The listing builds one solid part. Answer for the finished solid, in the listing's coordinates (mm). Give positions to 0.01 mm unless a question says otherwise; leave off trailing zeros. Order: outer loops, then holes, each group sorted by start corner. A loop starts at its lowest first (then second) coordinate and runs counter-clockwise, first axis right, second up. Notation, with made-up numbers: (43.25, 80) - (88.25, 80) arc R15 cw to (88.25, 95) - close; hole circle Ø6 at (-6, 14). An arc over 180 degrees is marked (long way). Use a Markdown table: item, result. Add a question column.
1) Straight lines are drawn through the part: line 1 (X direction, y = 1.75, z = 2.25); line 2 (Z direction, x = -20, y = 0.25); line 3 (Y direction, x = -0.5, z = -0.1). For each, find the intervals that lie inside material, in ascending order.
2) Find section A-A, the plane y = 13. Determine the outline of the cut face in (x, z).
3) Flat-ended cylindrical pins translate along their axes: pin 1 (0.9 mm diameter, centred on x = 15, z = 2, fed in from -Y); pin 2 (0.7 mm diameter, centred on y = 0, z = 2, fed in from +X); pin 3 (12 mm diameter, centred on x = -3, y = -4, fed in from +Z); pin 4 (1.5 mm diameter, centred on x = 11.5, z = 1, fed in from +Y). Find the tip coordinate at first contact, or state that the pin passes through.
4) Find section B-B, the plane x = -7. Determine the outline of the cut face in (y, z), plus the area to 3 significant figures.
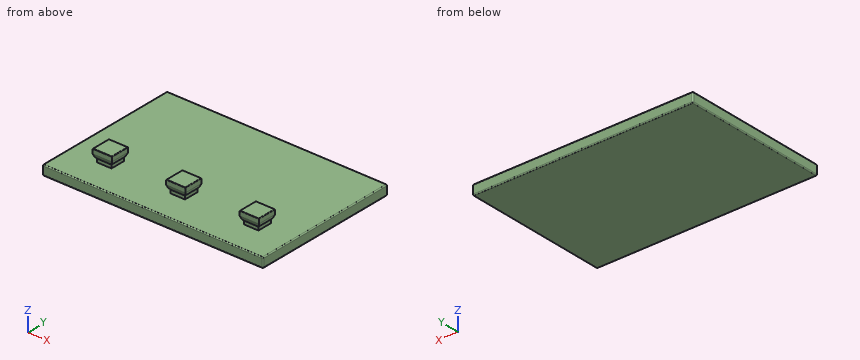
from build123d import *

# Parameters (mm, degrees)
SKETCH_1_W          = 45
SKETCH_1_H          = 30
EXTRUDE_1_DEPTH     = 2
SKETCH_2_W          = 3
SKETCH_2_H          = 3
EXTRUDE_2_DEPTH     = 1
EXTRUDE_START       = -4
EXTRUDE_3_DEPTH     = 5
CUT_EXTRUDE_1_REACH = 35.321
FILLET_1_R          = 0.1
FILLET_2_R          = 0.2


with BuildPart() as part:
    # Sketch 1 → Extrude 1 (new body)
    with BuildSketch(Plane.XY):
        with Locations((0, 7.5)):
            Rectangle(SKETCH_1_W, SKETCH_1_H)
    extrude(amount=-EXTRUDE_1_DEPTH)

    # Sketch 2 → Extrude 2 (add)
    with BuildSketch(Plane.XY):
        Rectangle(SKETCH_2_W, SKETCH_2_H)
    extrude_2 = extrude(amount=EXTRUDE_2_DEPTH)

    # Sketch 3 → Extrude 3 (add)
    with BuildSketch(Plane.XZ.offset(1.5).offset(EXTRUDE_START)):
        with BuildLine():
            Line((-1.95, 2.5), (1.95, 2.5))
            Line((1.95, 2.5), (1.95, 1.555590279))
            ThreePointArc((1.95, 1.555590279), (1.780042303, 1.088161527), (1.5, 0.677124344))
            Line((1.5, 0.677124344), (-1.5, 0.677124344))
            ThreePointArc((-1.5, 0.677124344), (-1.780042303, 1.088161527), (-1.95, 1.555590279))
            Line((-1.95, 1.555590279), (-1.95, 2.5))
        make_face()
    extrude_3 = extrude(amount=EXTRUDE_3_DEPTH)

    # Sketch 4 → Cut-Extrude 1 (cut, up to next)
    with BuildSketch(Plane.ZY.offset(1.95), mode=Mode.PRIVATE) as cut_extrude_1_sk1:
        with BuildLine():
            Line((0.677124344, 1.5), (0.677124344, 2.5))
            Line((0.677124344, 2.5), (2.5, 2.5))
            Line((2.5, 2.5), (2.5, 1.95))
            Line((2.5, 1.95), (1.555590279, 1.95))
            ThreePointArc((1.555590279, 1.95), (1.088161527, 1.780042303), (0.677124344, 1.5))
        make_face()
    cut_extrude_1_tool1 = extrude(cut_extrude_1_sk1.sketch, amount=-CUT_EXTRUDE_1_REACH, mode=Mode.PRIVATE) & part.part
    # Sketch 4 → Cut-Extrude 1 (cut, up to next)
    with BuildSketch(Plane.ZY.offset(1.95), mode=Mode.PRIVATE) as cut_extrude_1_sk2:
        with BuildLine():
            Line((0.677124344, -2.5), (2.5, -2.5))
            Line((2.5, -2.5), (2.5, -1.95))
            Line((2.5, -1.95), (1.555590279, -1.95))
            ThreePointArc((1.555590279, -1.95), (1.088161527, -1.780042303), (0.677124344, -1.5))
            Line((0.677124344, -1.5), (0.677124344, -2.5))
        make_face()
    cut_extrude_1_tool2 = extrude(cut_extrude_1_sk2.sketch, amount=-CUT_EXTRUDE_1_REACH, mode=Mode.PRIVATE) & part.part
    cut_extrude_1_1 = cut_extrude_1_tool1.solids().sort_by_distance((-1.95, 2.169375, 1.500125))[0]
    add(cut_extrude_1_1, mode=Mode.SUBTRACT)
    cut_extrude_1_2 = cut_extrude_1_tool2.solids().sort_by_distance((-1.95, -2.169375, 1.500125))[0]
    add(cut_extrude_1_2, mode=Mode.SUBTRACT)
    cut_extrude_1 = cut_extrude_1_1 + cut_extrude_1_2  # Cut-Extrude 1 as one shape, for the pattern or mirror that repeats it

    # Mirror 1: Extrude 2, Extrude 3, Cut-Extrude 1 across plane
    add(extrude_2.mirror(Plane(origin=(7.5, 0, 0), x_dir=(0, 0, 1), z_dir=(1, 0, 0))))
    add(extrude_3.mirror(Plane(origin=(7.5, 0, 0), x_dir=(0, 0, 1), z_dir=(1, 0, 0))))
    add(cut_extrude_1.mirror(Plane(origin=(7.5, 0, 0), x_dir=(0, 0, 1), z_dir=(1, 0, 0))), mode=Mode.SUBTRACT)

    # Mirror 2: Extrude 2, Extrude 3, Cut-Extrude 1 across plane
    add(extrude_2.mirror(Plane(origin=(-7.5, 0, 0), x_dir=(0, 0, 1), z_dir=(1, 0, 0))))
    add(extrude_3.mirror(Plane(origin=(-7.5, 0, 0), x_dir=(0, 0, 1), z_dir=(1, 0, 0))))
    add(cut_extrude_1.mirror(Plane(origin=(-7.5, 0, 0), x_dir=(0, 0, 1), z_dir=(1, 0, 0))), mode=Mode.SUBTRACT)

    # Fillet 1
    fillet_1_edges = [part.edges().sort_by_distance(p)[0] for p in [
        (15, -1.95, 2.5),
        (16.95, 0, 2.5),
        (13.05, 0, 2.5),
        (15, 1.95, 2.5),
        (-15, -1.95, 2.5),
        (-13.05, 0, 2.5),
        (-16.95, 0, 2.5),
        (-15, 1.95, 2.5),
        (0, -1.95, 2.5),
        (1.95, 0, 2.5),
        (-1.95, 0, 2.5),
        (0, 1.95, 2.5),
    ]]
    fillet(fillet_1_edges, radius=FILLET_1_R)

    # Fillet 2
    fillet_2_edges = [part.edges().sort_by_distance(p)[0] for p in [
        (22.5, 7.5, -2),
        (0, 22.5, -2),
        (-22.5, 7.5, -2),
        (0, 22.5, 0),
        (22.5, 7.5, 0),
        (0, -7.5, 0),
        (-22.5, 7.5, 0),
        (0, -7.5, -2),
        (-22.5, 22.5, -1),
        (22.5, 22.5, -1),
        (22.5, -7.5, -1),
        (-22.5, -7.5, -1),
    ]]
    fillet(fillet_2_edges, radius=FILLET_2_R)


solid = part.part
The answers:
| question | item | result |
|---|---|---|
| 1 | line 1 | -16.95 to -13.05, -1.95 to 1.95, 13.05 to 16.95 |
| 1 | line 2 | -2 to 0 |
| 1 | line 3 | -7.47 to 22.47 |
| 2 | outline | (-22.5, -1.8) arc R0.2 ccw to (-22.3, -2) - (22.3, -2) arc R0.2 ccw to (22.5, -1.8) - (22.5, -0.2) arc R0.2 ccw to (22.3, 0) - (-22.3, 0) arc R0.2 ccw to (-22.5, -0.2) - close |
| 3 | pin 1 | y = -1.95 |
| 3 | pin 2 | x = 16.95 |
| 3 | pin 3 | z = 2.5 |
| 3 | pin 4 | through |
| 4 | outline | (-7.5, -1.8) arc R0.2 ccw to (-7.3, -2) - (22.3, -2) arc R0.2 ccw to (22.5, -1.8) - (22.5, -0.2) arc R0.2 ccw to (22.3, 0) - (-7.3, 0) arc R0.2 ccw to (-7.5, -0.2) - close |
| 4 | area | 60.0 mm2 |
